Answer from the drawing. Dimensions are ordinates in mm from the lowest x, y and z of the part. Coordinates: 2 decimals unless noted, no trailing zeros. Write each loop counter-clockwise with the first axis right and the second up, starting at its lowest first coordinate (ties: lowest second). Pieces come first, ordered by that corner, then holes. Notation, with made-up numbers: (-15, 17.5) -> (36, 17.5) arc R31 cw to (36, 55.5) -> close; hole circle Ø7 at (50.25, 63.25). An arc over 180 degrees is marked (long way). Answer as a JSON object with one key per item and string values. Group by question number.
(1) Straight lines are drawn through the part: L1, parallel to X at y = 2.75, z = 5.25 (1 decimal); L2, parallel to X at y = 3.5, z = 14.75; L3, parallel to Y at x = 12, z = 13.5. For each, find the intervals that lie inside material, in ascending order.
(2) Flat-ended cylindrical pins translate along their axes: P1, Ø3, axis at y = 3.5, z = 13, coming from the +X side; P2, Ø5, axis at y = 5, z = 13.5, coming from the -X side; P3, Ø3, axis at x = 16.5, z = 3, coming from the -Y side. Find the tip coordinate at first contact, or state that the pin passes through.
(3) For a pull along X with two mould halves and no side action, classify the marked faces 1, 2 and 3 as +X half, -X half, draft (parallel to the pull), parting line (faces both ways), or undercut.
(4) Find section A-A (y = 8.75). Give the vertices of the cut face in (x, z).
(5) Find section B-B (y = 4). Give the vertices of the cut face in (x, z).
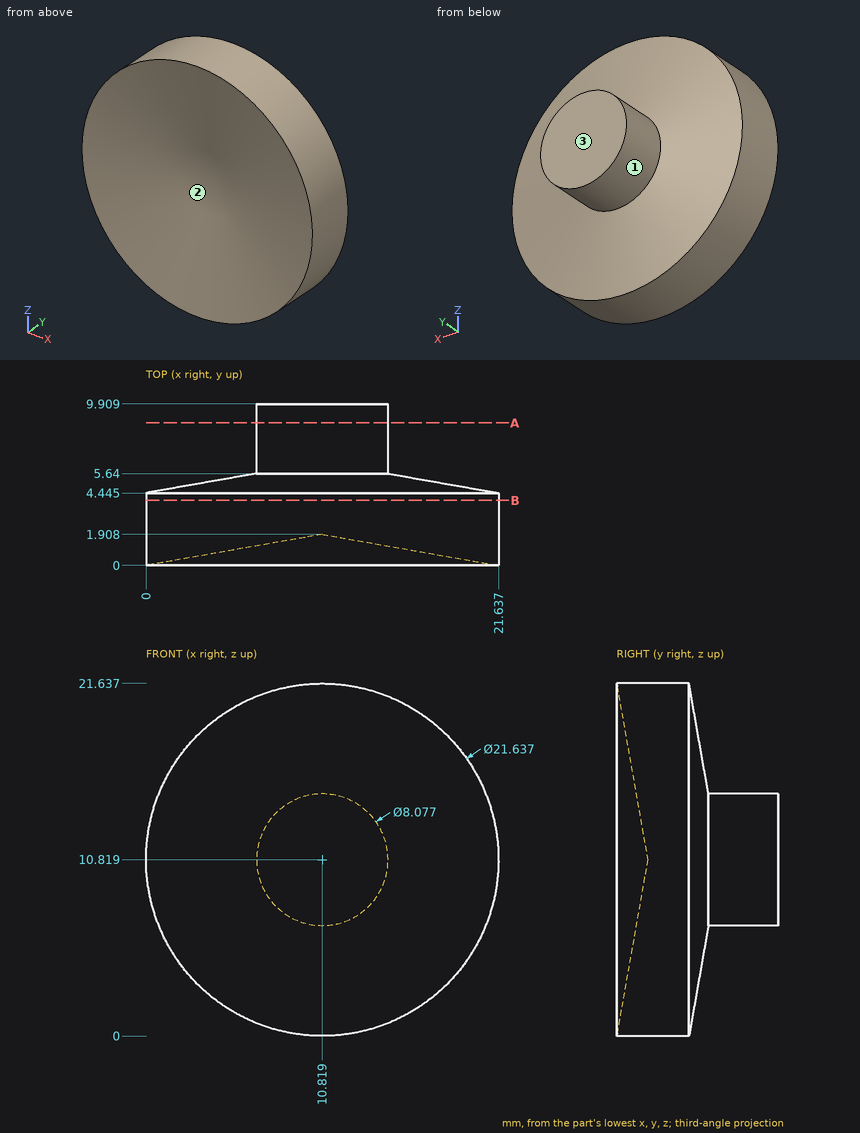
Results below:
{
 "1": {"L1": "x = 1.5 to 20.1", "L2": "x = 0.74 to 20.9", "L3": "y = 1.39 to 9.91"},
 "2": {"P1": "stops at x = 21.62", "P2": "stops at x = 0", "P3": "stops at y = 0"},
 "3": {"face 1": "parting line", "face 2": "undercut", "face 3": "draft"},
 "4": {"outline": "circle Ø8.08 at (10.82, 10.82)"},
 "5": {"outline": "circle Ø21.64 at (10.82, 10.82)"}
}
